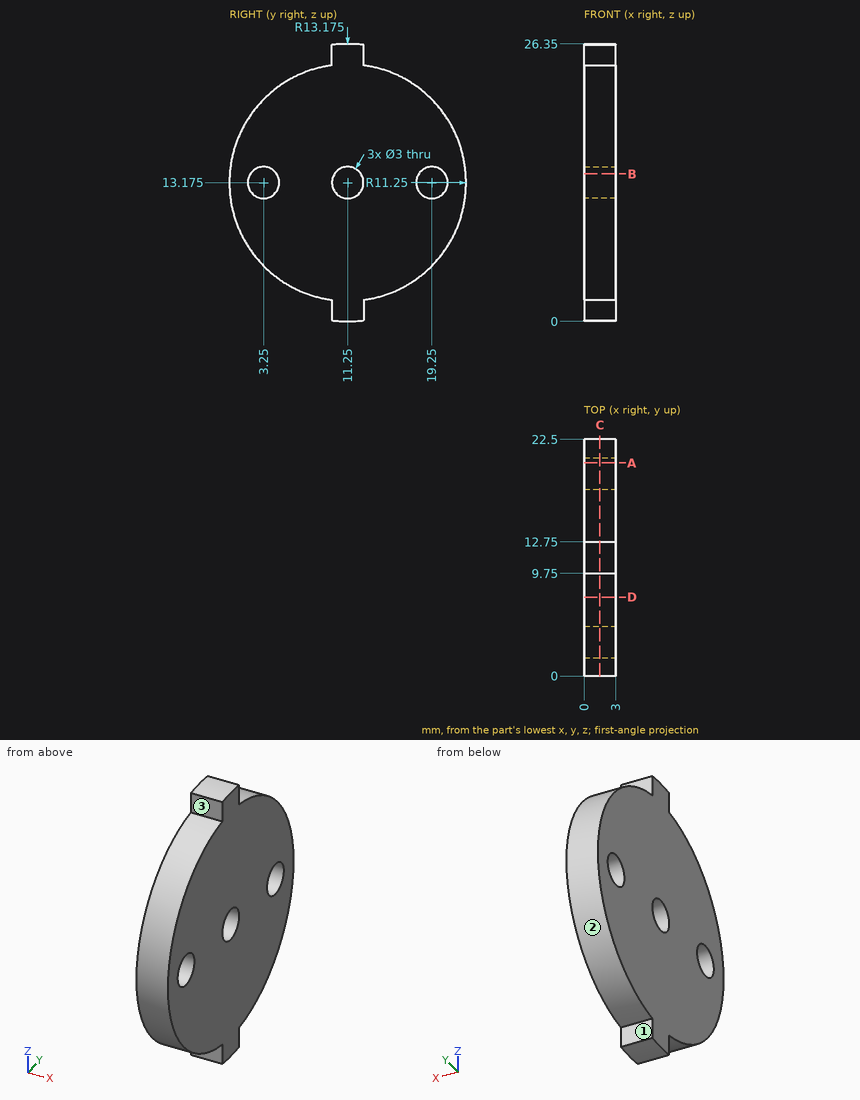
Job drawing, mm, ordinate dimensions from the low corner. One solid piece. A direction names the side the tool comes from. Give positions to 0.01 mm unless a question says otherwise; leave off trailing zeros. Write each loop counter-clockwise with the first axis right and the second up, starting at its lowest first coordinate (ties: lowest second). Pieces come first, ordered by that corner, then holes. Notation, with made-up numbers: (89, 78.5) -> (109, 78.5) arc R21 ccw to (109, 88.5) -> close; hole circle Ø4 at (21.25, -19). An arc over 180 degrees is marked (long way). Return JSON: item names as keys, results as strings.
Item 1: Band-saw the part on B-B (z = 14). List the corners of the cut face in (x, y).
Answer below:
{"outline": "(0, 0.03) -> (3, 0.03) -> (3, 2) -> (0, 2) -> close; (0, 4.5) -> (3, 4.5) -> (3, 10) -> (0, 10) -> close; (0, 12.5) -> (3, 12.5) -> (3, 18) -> (0, 18) -> close; (0, 20.5) -> (3, 20.5) -> (3, 22.47) -> (0, 22.47) -> close"}
Item 2: Drop flat-ended pins along their axis: pin 1 (1.8 mm diameter, centred on y = 11.25, z = 13.17, fed in from -X); pin 2 (1.6 mm diameter, centred on x = 1.5, z = 1, fed in from -Y); pin 3 (1 mm diameter, centred on x = 2.5, z = 4.5, fed in from +Y); pin 4 (1 mm diameter, centred on x = 1.5, z = 25, fed in from +Y). Give the stop position or say it passes through.
Answer below:
{"pin 1": "passes through", "pin 2": "stops at y = 9.75", "pin 3": "stops at y = 18.98", "pin 4": "stops at y = 12.75"}
Item 3: Tool access for the marked faces 1, 2 and 3: list every direction of +Z, -Z, +X, -X, +Y, -Y with a clear straight run to the whole face (end or side of a thin tool).
Answer below:
{"face 1": "-Z, +X, -X, +Y", "face 2": "+X, -X, +Y", "face 3": "+Z, +X, -X, -Y"}
Item 4: Band-saw the part on C-C (x = 1.5). Give the number of separate pieces and of enclosed holes in the cut face, then the cut area to 3 significant figures.
Answer below:
{"separate pieces": "1", "enclosed holes": "3", "area": "388 mm2"}
Item 5: Band-saw the part on D-D (y = 7.5). List the corners of the cut face in (x, z), then the cut area to 3 significant figures.
Answer below:
{"outline": "(0, 2.57) -> (3, 2.57) -> (3, 23.78) -> (0, 23.78) -> close", "area": "63.6 mm2"}
Item 6: Band-saw the part on A-A (y = 20.25). List the corners of the cut face in (x, z) (3 decimals), then the cut area to 3 significant figures.
Answer below:
{"outline": "(0, 6.425) -> (3, 6.425) -> (3, 12.057) -> (0, 12.057) -> close; (0, 14.293) -> (3, 14.293) -> (3, 19.925) -> (0, 19.925) -> close", "area": "33.8 mm2"}
Item 7: Drill centre lines: probe 1 along Y at (x, z) = (2.35, 12.5); probe 2 along Z at (x, y) = (1.85, 11.25) (3 decimals); probe 3 along Z at (x, y) = (1.4, 3). Where is each one in solid material? Low to high.
Answer below:
{"probe 1": "y = 0.02 to 1.91, 4.59 to 9.91, 12.59 to 17.91, 20.59 to 22.48", "probe 2": "z = 0 to 11.675, 14.675 to 26.35", "probe 3": "z = 5.53 to 11.7, 14.65 to 20.82"}
